Can you work these out from the model? Positions are in its coordinate system, mm. Give positions to 0.01 mm unless a question says otherwise; leave off trailing zeros. Write each loop counter-clockwise with the first axis right and the second up, starting at its lowest first coordinate (ties: lowest second). Pieces come first, ordered by that corner, then holes. Notation, with made-up numbers: M 14,89.25 L 49,89.25 A34 cw 49,128.25 Z; hole C -35.75,11.25 d9. An arc over 180 degrees is marked long. Write each question's results on one line, items separated by ' | '.
from build123d import *

# Parameters (mm, degrees)
SKETCH_1_R          = 12
SKETCH_1_R_2        = 1.5
SKETCH_1_R_3        = 6.3
EXTRUDE_1_DEPTH     = 3
EXTRUDE_2_DEPTH     = 3
FILLET_2_R          = 30
FILLET_4_R          = 1
SKETCH_3_R          = 1.5
CUT_EXTRUDE_1_DEPTH = 3
FILLET_6_R          = 3
SKETCH_5_R          = 2
EXTRUDE_3_DEPTH     = 3
FILLET_8_R          = 3
CUT_EXTRUDE_2_DEPTH = 10
EXTRUDE_4_DEPTH     = 3
CUT_EXTRUDE_4_DEPTH = 88.351282371
EXTRUDE_5_DEPTH     = 3
EXTRUDE_6_DEPTH     = 3
FILLET_9_R          = 10
FILLET_10_R         = 1
EXTRUDE_8_DEPTH     = 3
FILLET_11_R         = 5


with BuildPart() as part:
    # 草图1 → 凸台-拉伸1 (new body)
    with BuildSketch(Plane(origin=(0, 0, 0), x_dir=(0, 0, -1), z_dir=(1, 0, 0))):
        Circle(SKETCH_1_R)
        with Locations((0, 9)):
            Circle(SKETCH_1_R_2, mode=Mode.SUBTRACT)
        Circle(SKETCH_1_R_3, mode=Mode.SUBTRACT)
        with Locations((9, 0)):
            Circle(SKETCH_1_R_2, mode=Mode.SUBTRACT)
        with Locations((0, -9)):
            Circle(SKETCH_1_R_2, mode=Mode.SUBTRACT)
        with Locations((-9, 0)):
            Circle(SKETCH_1_R_2, mode=Mode.SUBTRACT)
    extrude(amount=EXTRUDE_1_DEPTH)

    # 草图4 → 凸台-拉伸2 (add)
    with BuildSketch(Plane.ZY):
        with BuildLine():
            Line((68.504845759, -22.032619578), (78, -30))
            Line((78, -30), (78, 3))
            Line((78, 3), (18.911534819, 13.41889066))
            Line((18.911534819, 13.41889066), (-0.877535827, 11.967870774))
            ThreePointArc((-0.877535827, 11.967870774), (8.169136125, 8.790063422), (12, 0))
            ThreePointArc((12, 0), (11.827182716, -2.029223745), (11.313708499, -4))
            Line((11.313708499, -4), (32.009040998, -6.929191455))
            Line((32.009040998, -6.929191455), (67.339599923, -4.571456898))
            Line((67.339599923, -4.571456898), (67.835333173, -12))
            Line((67.835333173, -12), (68.504845759, -22.032619578))
        make_face()
        Polygon((32.009040998, -6.929191455), (67.835333173, -12), (67.339599923, -4.571456898), align=None)
    extrude(amount=-EXTRUDE_2_DEPTH)

    # 圆角2
    fillet_2_edges = [part.edges().sort_by_distance(p)[0] for p in [
        (1.5, 13.41889066, 18.911534819),
    ]]
    fillet(fillet_2_edges, radius=FILLET_2_R)

    # 圆角4
    fillet_4_edges = [part.edges().sort_by_distance(p)[0] for p in [
        (1.5, -30, 78),
    ]]
    fillet(fillet_4_edges, radius=FILLET_4_R)

    # 草图3 → 切除-拉伸1 (cut)
    with BuildSketch(Plane.ZY):
        with Locations((50, 6)):
            Circle(SKETCH_3_R)
    extrude(amount=-CUT_EXTRUDE_1_DEPTH, mode=Mode.SUBTRACT)

    # 圆角6
    fillet_6_edges = [part.edges().sort_by_distance(p)[0] for p in [
        (1.5, -22.032619578, 68.504845759),
    ]]
    fillet(fillet_6_edges, radius=FILLET_6_R)

    # 草图5 → 凸台-拉伸3 (add)
    with BuildSketch(Plane(origin=(3, 0, 0), x_dir=(0, 0, -1), z_dir=(1, 0, 0))):
        with BuildLine():
            Line((11.833611983, 1.991388321), (8.212146403, 23.511559971))
            ThreePointArc((8.212146403, 23.511559971), (6.010394905, 26.448138505), (2.341304536, 26.353380903))
            Line((2.341304536, 26.353380903), (-22.28242614, 12.822865834))
            Line((-22.28242614, 12.822865834), (0.877535827, 11.967870774))
            Line((0.877535827, 11.967870774), (11.833611983, 1.991388321))
        make_face()
        with Locations((3.76079209, 21.676172237)):
            Circle(SKETCH_5_R, mode=Mode.SUBTRACT)
    extrude(amount=-EXTRUDE_3_DEPTH)

    # 圆角8
    fillet_8_edges = [part.edges().sort_by_distance(p)[0] for p in [
        (1.5, 12.822865834, 22.28242614),
    ]]
    fillet(fillet_8_edges, radius=FILLET_8_R)

    # 草图6 → 切除-拉伸2 (cut)
    with BuildSketch(Plane(origin=(3, 0, 0), x_dir=(0, 0, -1), z_dir=(1, 0, 0))):
        with BuildLine():
            ThreePointArc((-11.313708499, -4), (-11.827182716, -2.029223745), (-12, 0))
            Line((-12, 0), (-67.835333173, -6))
            Line((-67.835333173, -6), (-67.835333173, -12))
            Line((-67.835333173, -12), (-11.313708499, -4))
        make_face()
    extrude(amount=-CUT_EXTRUDE_2_DEPTH, mode=Mode.SUBTRACT)

    # 草图7 → 凸台-拉伸4 (add)
    with BuildSketch(Plane(origin=(3, 0, 0), x_dir=(0, 0, -1), z_dir=(1, 0, 0))):
        with BuildLine():
            ThreePointArc((-76.35721239, -28.621537523), (-77.422618262, -28.761800867), (-78, -27.855493079))
            Line((-78, -27.855493079), (-78, -39.207735307))
            Line((-78, -39.207735307), (-65.698458682, -28.885516524))
            Line((-65.698458682, -28.885516524), (-67.835333173, -9))
            Line((-67.835333173, -9), (-67.835333173, -12))
            Line((-67.835333173, -12), (-68.419679282, -20.756403294))
            ThreePointArc((-68.419679282, -20.756403294), (-68.737840819, -21.914368693), (-69.484658626, -22.854780194))
            Line((-69.484658626, -22.854780194), (-76.35721239, -28.621537523))
        make_face()
    extrude(amount=-EXTRUDE_4_DEPTH)

    # 草图9 → 切除-拉伸4 (cut, through all)
    with BuildSketch(Plane(origin=(3, 0, 0), x_dir=(0, 0, -1), z_dir=(1, 0, 0))):
        Polygon((-51.477915802, -4.242250943), (-102.730700366, -9.749815596), (-98.933525576, -45.085902185), (-47.680741012, -39.578337532), align=None)
    extrude(amount=-CUT_EXTRUDE_4_DEPTH, mode=Mode.SUBTRACT)

    # 草图10 → 凸台-拉伸5 (add)
    with BuildSketch(Plane.ZY):
        Polygon((78, -7.092283282), (93, -8.704165846), (93, 0.355095289), (78, 3), align=None)
    extrude(amount=-EXTRUDE_5_DEPTH)

    # 草图11 → 凸台-拉伸6 (add)
    with BuildSketch(Plane.ZY):
        Polygon((93, -8.704165846), (85.276239998, -47.951376338), (78.172649999, -32.159084028), (83, -7.62957747), align=None)
    extrude(amount=-EXTRUDE_6_DEPTH)

    # 圆角9
    fillet_9_edges = [part.edges().sort_by_distance(p)[0] for p in [
        (1.5, 0.355095289, 93),
        (1.5, -32.159084028, 78.172649999),
        (1.5, -7.62957747, 83),
    ]]
    fillet(fillet_9_edges, radius=FILLET_9_R)

    # 圆角10
    fillet_10_edges = [part.edges().sort_by_distance(p)[0] for p in [
        (1.5, -47.951376338, 85.276239998),
    ]]
    fillet(fillet_10_edges, radius=FILLET_10_R)

    # 草图12 → 凸台-拉伸8 (add)
    with BuildSketch(Plane(origin=(3, 0, 0), x_dir=(0, 0, -1), z_dir=(1, 0, 0))):
        with BuildLine():
            Line((3.180339281, 26.697159193), (-85.718174485, 1.587587299))
            ThreePointArc((-85.718174485, 1.587587299), (-85.230157098, 1.712247485), (-84.736481777, 1.812176508))
            Line((-84.736481777, 1.812176508), (-22.766810048, 12.739101619))
            ThreePointArc((-22.766810048, 12.739101619), (-22.291557819, 12.863755981), (-21.843026177, 13.064312099))
            Line((-21.843026177, 13.064312099), (2.341304536, 26.353380903))
            ThreePointArc((2.341304536, 26.353380903), (2.751049335, 26.549121258), (3.180339281, 26.697159193))
        make_face()
    extrude(amount=-EXTRUDE_8_DEPTH)

    # 圆角11
    fillet_11_edges = [part.edges().sort_by_distance(p)[0] for p in [
        (1.5, 0, 12),
    ]]
    fillet(fillet_11_edges, radius=FILLET_11_R)


solid = part.part
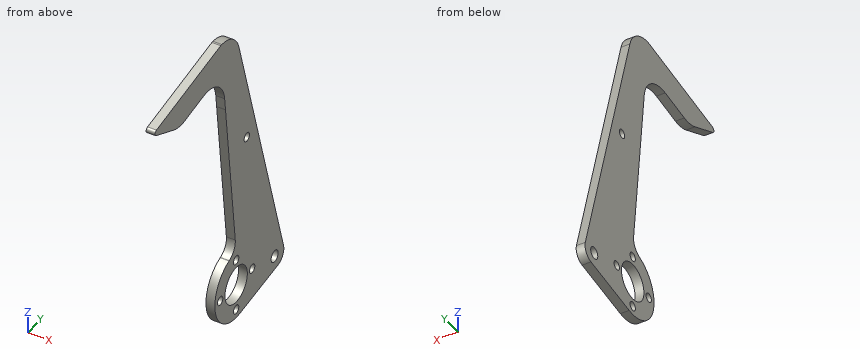
Item 1: I want a section at D-D, the plane z = 53. Please give me the cut outline in (x, y).
Geometry says:
outline: M 0,-4.41 L 3,-4.41 L 3,10.83 L 0,10.83 Z
Item 2: I want a section at A-A, the plane z = 9. Please give me the cut outline in (x, y), and give its area (3 significant figures).
Geometry says:
outline: M 0,-7.94 L 3,-7.94 L 3,-1.5 L 0,-1.5 Z; M 0,1.5 L 3,1.5 L 3,23.26 L 0,23.26 Z | area: 84.6 mm2
Item 3: I want a section at B-B, the plane x = 0.75. Please give me the cut outline in (y, z), and give its area (3 significant figures).
Geometry says:
outline: M -45.09,83.99 L -35.07,79.48 A10 ccw -29.03,78.79 L -18.34,80.89 A10 cw -6.46,72.15 L -0.5,16.63 A5 cw -3.86,11.36 A12 ccw 1.99,-11.83 L 23.51,-8.21 A4 ccw 26.7,-3.18 L 1.59,85.72 A10 ccw -8.04,93 L -8.7,93 L -44.87,85.88 A1 ccw Z; hole C -9,0 d3; hole C 0,0 d12.6; hole C 0,-9 d3; hole C 0,9 d3; hole C 6,50 d3; hole C 9,0 d3; hole C 21.68,-3.76 d4 | area: 2,190 mm2
Item 4: I want a section at C-C, the plane y = 17.5. Please give me the cut outline in (x, z), and give its area (3 significant figures).
Geometry says:
outline: M 0,-9.22 L 3,-9.22 L 3,29.38 L 0,29.38 Z | area: 116 mm2
Item 5: I'm going to push flat-ended pins straight in: pin 1 (1 mm diameter, centred on x = 2.5, z = 61, fed in from +Y); pin 2 (1.8 mm diameter, centred on y = 0, z = 9, fed in from +X); pin 3 (1.5 mm diameter, centred on x = 1, z = 19.5, fed in from +Y). Where does each tip first touch, or does it pass through?
Geometry says:
pin 1: stops at y = 8.71 | pin 2: passes through | pin 3: stops at y = 20.5
Item 6: If I drill on line 1 (Y direction, x = 0.4, z = -4); line 2 (Y direction, x = 2.55, z = 74.5); line 3 (Z direction, x = 2.25, y = -43), over which ranges is the centre line in solid material (lowest first)? Write a range as from..to.
Geometry says:
line 1: y = -11.31..-4.87, 4.87..19.69, 23.66..26.84 | line 2: y = -7.01..4.76 | line 3: z = 83.05..86.25
